Autodesk Inventor part; units mm, degrees
ref_plane "YZ Plane" through (0, 0, 0) normal (1, 0, 0) x (0, 1, 0)
ref_plane "XZ Plane" through (0, 0, 0) normal (0, 1, 0) x (-1, 0, 0)
ref_plane "XY Plane" through (0, 0, 0) normal (0, 0, 1) x (1, 0, 0)
sketch "Sketch1" plane through (0, 0, 0) normal (0, 1, 0) x (-1, 0, 0)
  circle A0 centre (0, 0) radius 14.05
  circle A1 centre (0, 0) radius 19.55 construction
  circle A2 centre (0, -22.55) radius 1.95
  circle A3 centre (0, 22.55) radius 1.95
  circle A4 centre (0, 22.55) radius 4.95 construction
  circle A5 centre (0, -22.55) radius 4.95 construction
  line L0 (19.55, 27.5) -> (-19.55, 27.5) construction
  line L1 (-19.55, 27.5) -> (-19.55, -27.5) construction
  line L2 (-19.55, -27.5) -> (19.55, -27.5) construction
  line L3 (19.55, -27.5) -> (19.55, 27.5) construction
  line L4 (0, 22.55) -> (0, -22.55) construction
  line L5 (-22.55, 30.5) -> (22.55, 30.5)
  line L6 (22.55, 30.5) -> (22.55, -30.5)
  line L7 (22.55, -30.5) -> (-22.55, -30.5)
  line L8 (-22.55, -30.5) -> (-22.55, 30.5)
  dimension "d0" = 28.1
  dimension "d1" = 5.5
  dimension "d2" = 3.9
  dimension "d3" = 3.9
  dimension "d4" = 22.55
  dimension "d5" = 22.55
  dimension "d6" = 3
  dimension "d7" = 3
  dimension "d8" = 3
extrude "Extrusion1" add sketch "Sketch1" along normal blind 3
equation "\"d5\" = d4"
properties part number "10p_passthrough_profile"
Geometry check sheet. Reference: the model listing, model coordinates, mm. Give positions to 0.01 mm unless a question says otherwise; leave off trailing zeros. Order: outer loops, then holes, each group sorted by start corner. A loop starts at its lowest first (then second) coordinate and runs counter-clockwise, first axis right, second up. Notation, with made-up numbers: (-29.75, 37.5) - (-7.75, 37.5) arc R17 ccw to (-7.75, 58.5) - close; hole circle Ø7 at (33, -24.75). An arc over 180 degrees is marked (long way). Answer as a JSON object with one key per item and string values.
(1) Draft check along X on faces 1 (the flat face through (-22.55, 1, 0)), 2 (the flat face through (0, 1, -30.5)), 3 (the cylindrical face through (3.046, 1.479, 13.716)). Enter one of: released by +X, released by -X, zero draft, split by the parting line, or undercut.
Report:
{"face 1": "released by -X", "face 2": "zero draft", "face 3": "undercut"}
(2) Material ranges on line 1 (Z direction, x = 0, y = 0.8); line 2 (X direction, y = 2.15, z = 0.5); line 3 (Z direction, x = 10.5, y = 0.35), recorded low to high.
Report:
{"line 1": "-30.5 to -24.5, -20.6 to -14.05, 14.05 to 20.6, 24.5 to 30.5", "line 2": "-22.55 to -14.04, 14.04 to 22.55", "line 3": "-30.5 to -9.34, 9.34 to 30.5"}
(3) Cross-section at D-D (x = 7.5). Record the cut outline in (y, z).
Report:
{"outline": "(0, -30.5) - (3, -30.5) - (3, -11.88) - (0, -11.88) - close; (0, 11.88) - (3, 11.88) - (3, 30.5) - (0, 30.5) - close"}
(4) Cross-section at A-A (z = 0). Record the cut outline in (x, y).
Report:
{"outline": "(-22.55, 0) - (-14.05, 0) - (-14.05, 3) - (-22.55, 3) - close; (14.05, 0) - (22.55, 0) - (22.55, 3) - (14.05, 3) - close"}
(5) Cross-section at C-C (y = 1.8). Record the cut outline in (x, z).
Report:
{"outline": "(-22.55, -30.5) - (22.55, -30.5) - (22.55, 30.5) - (-22.55, 30.5) - close; hole circle Ø28.1 at (0, 0); hole circle Ø3.9 at (0, -22.55); hole circle Ø3.9 at (0, 22.55)"}
(6) Depth check by flat-ended pin: pin 1 Ø3 at (x, z) = (0, -22.55) entering from -Y (3 decimals). Enter the tip coordinate at first touch or a pass-through.
Report:
{"pin 1": "through"}
(7) Cross-section at B-B (x = 0). Record the cut outline in (y, z).
Report:
{"outline": "(0, -30.5) - (3, -30.5) - (3, -24.5) - (0, -24.5) - close; (0, -20.6) - (3, -20.6) - (3, -14.05) - (0, -14.05) - close; (0, 14.05) - (3, 14.05) - (3, 20.6) - (0, 20.6) - close; (0, 24.5) - (3, 24.5) - (3, 30.5) - (0, 30.5) - close"}
